Geometry: final body of the model. Coordinates: model frame, mm. Face numbers are marked on the shaded views. Give positions to 0.01 mm unless a question says otherwise; leave off trailing zeros. Write each loop counter-clockwise with the first axis right and the second up, starting at its lowest first coordinate (ties: lowest second). Pieces come first, ordered by that corner, then holes. Notation, with made-up numbers: M 35,76 L 94,76 A8 cw 94,87 Z; hole C 80.25,11 d2. An arc over 180 degrees is marked long. Use a Markdown table: item, result. Add a question column.
1) Line query: line 1 (X direction, y = 10, z = 2.1); line 2 (X direction, y = 9, z = 0.7). Output: solid intervals per line, ascending.
2) Section D-D on x = 10. Return the cut outline in (y, z).
3) Draft query along X for the marked faces 1, 2 and 3. Return one class per face: +X half, -X half, draft (parallel to the pull), parting line (faces both ways), or undercut.
4) Section A-A on x = 60. Return the cut outline in (y, z).
5) Section C-C on z = 1.9. Return the cut outline in (x, y).
6) Pin query (flat end, axial travel): pin 1 (1 mm diameter, centred on x = 41, z = 0.5, fed in from +Y); pin 2 (4.5 mm diameter, centred on x = 10, y = 35, fed in from -Z); pin 3 (1 mm diameter, centred on y = 40, z = 1, fed in from +X); pin 4 (1 mm diameter, centred on x = 8, z = 1.5, fed in from -Y). Return the tip coordinate at first contact, or that it passes through.
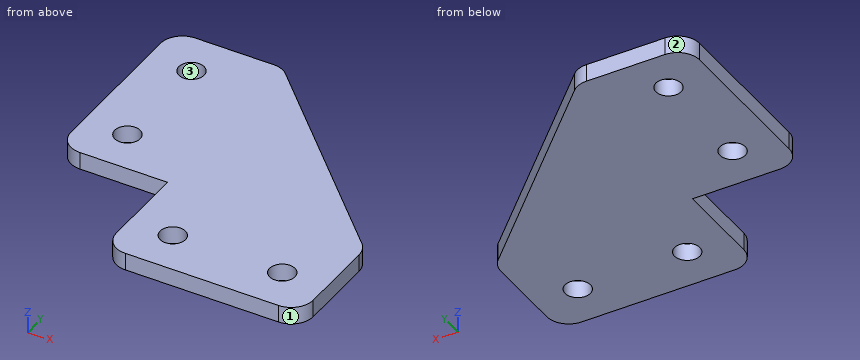
Autodesk Fusion 360 part; units mm, degrees
sketch "Bracket Shape" plane through (0, 0, 0) normal (0, 0, 1) x (1, 0, 0) in component "Bracket"
  line L0 (0, 0) -> (70, 0)
  line L1 (70, 0) -> (70, 70)
  line L2 (70, 70) -> (0, 70)
  line L3 (0, 70) -> (0, 0)
  line L4 (0, 0) -> (25, 0)
  line L5 (25, 0) -> (25, 25)
  line L6 (25, 25) -> (0, 25)
  line L7 (0, 25) -> (0, 0)
  line L8 (25, 25) -> (25, 70)
  line L9 (25, 25) -> (70, 25)
  line L10 (25, 70) -> (70, 25)
  line L11 (0, 70) -> (10, 70)
  line L12 (10, 70) -> (10, 25) construction
  line L13 (70, 0) -> (70, 10) construction
  line L14 (70, 10) -> (25, 10) construction
  line L15 (70, 0) -> (60, 0) construction
  line L16 (25, 0) -> (35, 0) construction
  line L17 (35, 0) -> (35, 10) construction
  line L18 (60, 0) -> (60, 10) construction
  line L19 (0, 25) -> (0, 35) construction
  line L20 (0, 70) -> (0, 60) construction
  line L21 (0, 70) -> (0, 60) construction
  line L22 (0, 35) -> (10, 35) construction
  line L23 (0, 60) -> (10, 60) construction
  line L24 (25, 10) -> (0, 10) construction
  line L25 (10, 25) -> (10, 0) construction
  dimension "d1" = 70
  dimension "d2" = 70
  dimension "d3" = 25
  dimension "d4" = 25
  dimension "d7" = 10
  dimension "d8" = 10
  dimension "d9" = 10
  dimension "d10" = 10
  dimension "d11" = 10
  dimension "d12" = 10
extrude "Extrude1" add sketch "Bracket Shape" along normal blind 4 contours L0 L1 L5 L9 | L2 L3 L6 L8 L11 | L8 L9 L10 in component "Bracket"
hole "Hole1" at (10, 60, 0) direction (0, 0, 1) diameter 5.8 end through all in component "Bracket"
hole "Hole2" at (10, 35, 0) direction (0, 0, 1) diameter 5.8 end through all in component "Bracket"
hole "Hole3" at (35, 10, 0) direction (0, 0, 1) diameter 5.8 end through all in component "Bracket"
hole "Hole4" at (60, 10, 0) direction (0, 0, 1) diameter 5.8 end through all in component "Bracket"
fillet "Fillet1" radius 5 6 edges at (70, 0, 2) (25, 0, 2) (0, 25, 2) (0, 70, 2) (25, 70, 2) (70, 25, 2) in component "Bracket"
component "Bracket" placed x (1, 0, 0) y (0, 1, 0) z (0, 0, 1) at (0, 0, 0)
Found:
| question | item | result |
|---|---|---|
| 1 | line 1 | 25 to 32.1, 37.9 to 57.1, 62.9 to 70 |
| 1 | line 2 | 25 to 32.28, 37.72 to 57.28, 62.72 to 70 |
| 2 | outline | M 25,0 L 32.1,0 L 32.1,4 L 25,4 Z; M 37.9,0 L 57.1,0 L 57.1,4 L 37.9,4 Z; M 62.9,0 L 70,0 L 70,4 L 62.9,4 Z |
| 3 | face 1 | +X half |
| 3 | face 2 | -X half |
| 3 | face 3 | undercut |
| 4 | outline | M 0,0 L 7.1,0 L 7.1,4 L 0,4 Z; M 12.9,0 L 35,0 L 35,4 L 12.9,4 Z |
| 5 | outline | M 0,30 A5 ccw 5,25 L 25,25 L 25,5 A5 ccw 30,0 L 65,0 A5 ccw 70,5 L 70,22.93 A5 ccw 68.54,26.46 L 26.46,68.54 A5 ccw 22.93,70 L 5,70 A5 ccw 0,65 Z; hole C 10,35 d5.8; hole C 10,60 d5.8; hole C 35,10 d5.8; hole C 60,10 d5.8 |
| 6 | pin 1 | y = 54.5 |
| 6 | pin 2 | through |
| 6 | pin 3 | x = 55.5 |
| 6 | pin 4 | y = 25 |
